Answer from the drawing. Dimensions are ordinates in mm from the lowest x, y and z of the part. Round coordinates to 2 decimals unless told otherwise and drop trailing zeros. Loops run counter-clockwise (first coordinate to the right, second up) from the corner with the lowest first, then second, coordinate; pieces in that order, holes last. Notation, with made-up numbers: M 44,4 L 82,4 A30 cw 82,39 Z; hole C -26,6 d4. An arc over 180 degrees is marked long. One line per item, written item: value.
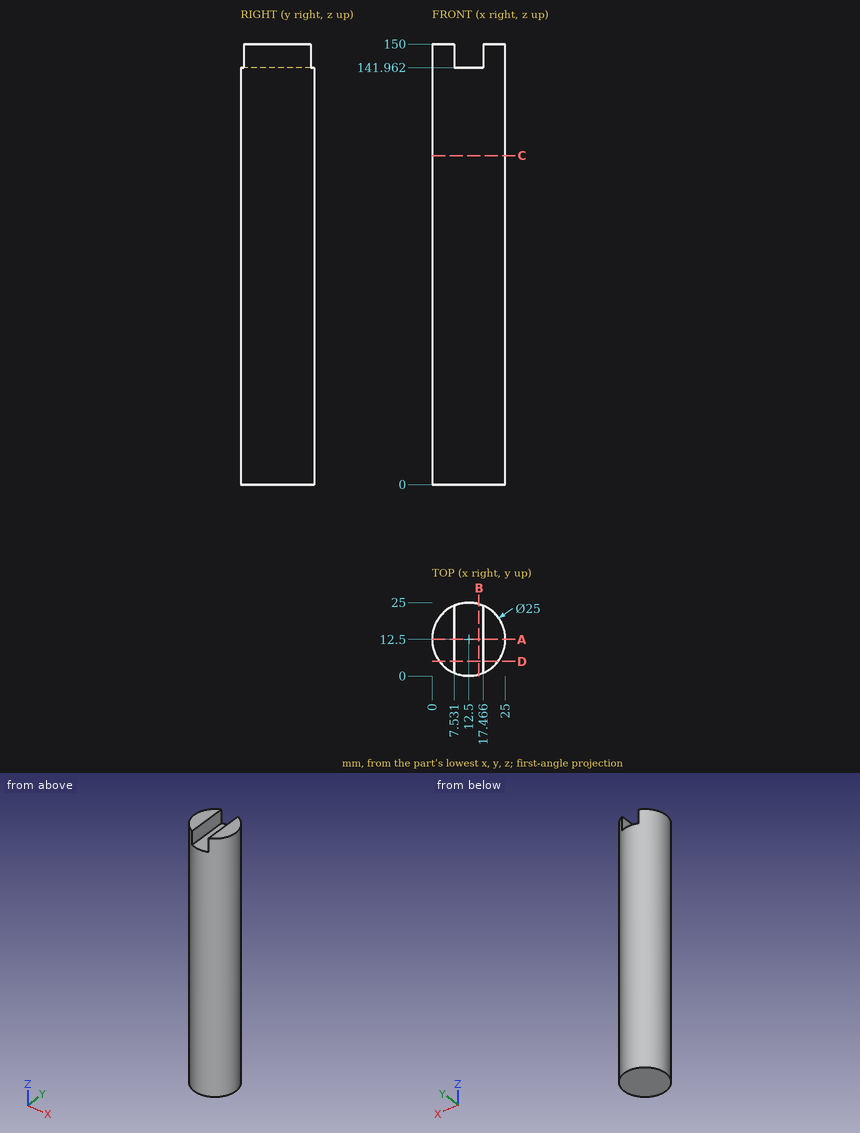
1) Each of these flat-tipped pins is pushed along its axis until it touches: pin 1 (8 mm diameter, centred on x = 9.5, y = 13, fed in from +Z); pin 2 (5 mm diameter, centred on x = 19, z = 86, fed in from -Y); pin 3 (12 mm diameter, centred on y = 4, z = 30.5, fed in from -X); pin 4 (6 mm diameter, centred on x = 5, z = 131.5, fed in from +Y). Where does it stop, or does it pass through?
Check values:
pin 1: z = 150
pin 2: y = 0.66
pin 3: x = 0.25
pin 4: y = 24.16
2) Find section B-B (x = 16). Give the vertices of the cut face in (y, z), then the cut area to 3 significant figures.
Check values:
outline: M 0.5,0 L 24.5,0 L 24.5,141.96 L 0.5,141.96 Z
area: 3,410 mm2
3) Find the intervals of material crossed by probe 1 along Z at (x, y) = (11, 20.75); probe 2 along X at (y, z) = (7.5, 12.5) (1 decimal); probe 3 along Y at (x, z) = (13.25, 56), in increasing order. Write a range as from..to.
Check values:
probe 1: 0..141.96
probe 2: 1..24
probe 3: 0.02..24.98
4) Find section A-A (y = 12.5). Give the vertices of the cut face in (x, z) (1 decimal), then the cut area to 3 significant figures.
Check values:
outline: M 0,0 L 25,0 L 25,150 L 17.5,150 L 17.5,142 L 7.5,142 L 7.5,150 L 0,150 Z
area: 3,670 mm2
5) Find section C-C (z = 112). Give the vertices of the cut face in (x, y), then the cut area to 3 significant figures.
Check values:
outline: C 12.5,12.5 d25
area: 491 mm2
6) Find section D-D (y = 5). Give the vertices of the cut face in (x, z) (1 decimal), then the cut area to 3 significant figures.
Check values:
outline: M 2.5,0 L 22.5,0 L 22.5,150 L 17.5,150 L 17.5,142 L 7.5,142 L 7.5,150 L 2.5,150 Z
area: 2,920 mm2
